from build123d import *

# Parameters (mm, degrees)
EXTRUDE_1_DEPTH     = 2
CUT_EXTRUDE_1_DEPTH = 15.604642381
EXTRUDE_START       = -1.63
EXTRUDE_2_DEPTH     = 1.63
CUT_EXTRUDE_2_DEPTH = 1.2
CUT_EXTRUDE_3_DEPTH = 0.37
FILLET_3_R          = 1.2


with BuildPart() as part:
    # 草图1 → 凸台-拉伸1 (new body)
    with BuildSketch(Plane(origin=(0, 0, 0), x_dir=(-1, 0, 0), z_dir=(0, 1, 0))):
        with BuildLine():
            Line((7.77, 10.437594514), (-7.77, 10.437594514))
            ThreePointArc((-7.77, 10.437594514), (-9.359289322, 9.779289322), (-10.017594514, 8.19))
            Line((-10.017594514, 8.19), (-10.017594514, -8.19))
            ThreePointArc((-10.017594514, -8.19), (-9.359289322, -9.779289322), (-7.77, -10.437594514))
            Line((-7.77, -10.437594514), (7.77, -10.437594514))
            ThreePointArc((7.77, -10.437594514), (9.359289322, -9.779289322), (10.017594514, -8.19))
            Line((10.017594514, -8.19), (10.017594514, 8.19))
            ThreePointArc((10.017594514, 8.19), (9.359289322, 9.779289322), (7.77, 10.437594514))
        make_face()
    extrude(amount=EXTRUDE_1_DEPTH)

    # 草图3 → 切除-拉伸1 (cut, through all)
    with BuildSketch(Plane(origin=(0, 2, 0), x_dir=(1, 0, 0), z_dir=(0, 1, 0))):
        with BuildLine():
            Line((3.175, 8.940777212), (-3.175, 8.940777212))
            ThreePointArc((-3.175, 8.940777212), (-4.200304833, 8.516082045), (-4.625, 7.490777212))
            Line((-4.625, 7.490777212), (-4.625, 6.930777212))
            ThreePointArc((-4.625, 6.930777212), (-4.200304833, 5.90547238), (-3.175, 5.480777212))
            Line((-3.175, 5.480777212), (3.175, 5.480777212))
            ThreePointArc((3.175, 5.480777212), (4.200304833, 5.90547238), (4.625, 6.930777212))
            Line((4.625, 6.930777212), (4.625, 7.490777212))
            ThreePointArc((4.625, 7.490777212), (4.200304833, 8.516082045), (3.175, 8.940777212))
        make_face()
    extrude(amount=-CUT_EXTRUDE_1_DEPTH, mode=Mode.SUBTRACT)

    # 草图4 → 凸台-拉伸2 (add)
    with BuildSketch(Plane.XZ.offset(EXTRUDE_START)):
        with BuildLine():
            Line((-4.625, -7.490777212), (-4.625, -6.930777212))
            ThreePointArc((-4.625, -6.930777212), (-4.200304833, -5.90547238), (-3.175, -5.480777212))
            Line((-3.175, -5.480777212), (3.175, -5.480777212))
            ThreePointArc((3.175, -5.480777212), (4.200304833, -5.90547238), (4.625, -6.930777212))
            Line((4.625, -6.930777212), (4.625, -7.490777212))
            ThreePointArc((4.625, -7.490777212), (4.200304833, -8.516082045), (3.175, -8.940777212))
            Line((3.175, -8.940777212), (-3.175, -8.940777212))
            ThreePointArc((-3.175, -8.940777212), (-4.200304833, -8.516082045), (-4.625, -7.490777212))
        make_face()
        with BuildLine():
            Line((3.175, -8.540777212), (-3.175, -8.540777212))
            ThreePointArc((-3.175, -8.540777212), (-3.91746212, -8.233239333), (-4.225, -7.490777212))
            Line((-4.225, -7.490777212), (-4.225, -6.930777212))
            ThreePointArc((-4.225, -6.930777212), (-3.91746212, -6.188315092), (-3.175, -5.880777212))
            Line((-3.175, -5.880777212), (3.175, -5.880777212))
            ThreePointArc((3.175, -5.880777212), (3.91746212, -6.188315092), (4.225, -6.930777212))
            Line((4.225, -6.930777212), (4.225, -7.490777212))
            ThreePointArc((4.225, -7.490777212), (3.91746212, -8.233239333), (3.175, -8.540777212))
        make_face(mode=Mode.SUBTRACT)
    extrude(amount=EXTRUDE_2_DEPTH)

    # 草图5 → 切除-拉伸2 (cut)
    with BuildSketch(Plane(origin=(0, 2, 0), x_dir=(1, 0, 0), z_dir=(0, 1, 0))):
        with BuildLine():
            Line((9.417594514, 4.880777212), (-9.417594514, 4.880777212))
            Line((-9.417594514, 4.880777212), (-9.417594514, -8.19))
            ThreePointArc((-9.417594514, -8.19), (-8.935025253, -9.355025253), (-7.77, -9.837594514))
            Line((-7.77, -9.837594514), (7.77, -9.837594514))
            ThreePointArc((7.77, -9.837594514), (8.935025253, -9.355025253), (9.417594514, -8.19))
            Line((9.417594514, -8.19), (9.417594514, 4.880777212))
        make_face()
    extrude(amount=-CUT_EXTRUDE_2_DEPTH, mode=Mode.SUBTRACT)

    # 草图7 → 切除-拉伸3 (cut)
    with BuildSketch(Plane(origin=(0, 2, 0), x_dir=(1, 0, 0), z_dir=(0, 1, 0))):
        with BuildLine():
            Line((9.417594514, 8.19), (9.417594514, 4.880777212))
            Line((9.417594514, 4.880777212), (-9.417594514, 4.880777212))
            Line((-9.417594514, 4.880777212), (-9.417594514, 8.19))
            ThreePointArc((-9.417594514, 8.19), (-8.935025253, 9.355025253), (-7.77, 9.837594514))
            Line((-7.77, 9.837594514), (7.77, 9.837594514))
            ThreePointArc((7.77, 9.837594514), (8.935025253, 9.355025253), (9.417594514, 8.19))
        make_face()
    extrude(amount=-CUT_EXTRUDE_3_DEPTH, mode=Mode.SUBTRACT)

    # 圆角3
    fillet_3_edges = [part.edges().sort_by_distance(p)[0] for p in [
        (9.417594514, 1.215, -4.880777212),
        (-9.417594514, 1.215, -4.880777212),
    ]]
    fillet(fillet_3_edges, radius=FILLET_3_R)


solid = part.part
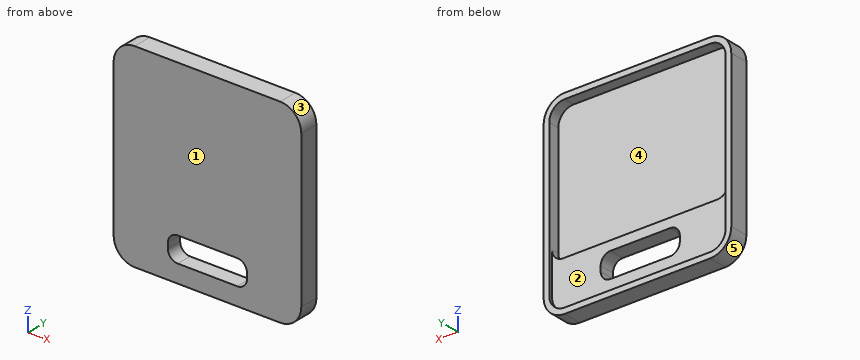
Work out the finished part from the listing and answer in its coordinate system (mm). Face numbers are marked on the shaded views. A direction names the side the tool comes from. Give positions to 0.01 mm unless a question says otherwise; leave off trailing zeros. Loops run counter-clockwise (first coordinate to the right, second up) from the corner with the lowest first, then second, coordinate; pieces in that order, holes last. Notation, with made-up numbers: (32.25, -14.5) - (45.25, -14.5) arc R20 ccw to (45.25, 1.5) - close; hole circle Ø6 at (8.5, 75). An arc over 180 degrees is marked (long way). Answer in a Markdown table with one row per item.
(1) Section C-C (z = -7.75) is taken. Give the vertices of the cut face in (x, y), and give its area (3 significant figures).
Results list:
| item | result |
|---|---|
| outline | (-10.02, 0) - (-4.19, 0) - (-4.19, 1.63) - (-9.42, 1.63) - (-9.42, 2) - (-10.02, 2) - close; (4.19, 0) - (10.02, 0) - (10.02, 2) - (9.42, 2) - (9.42, 1.63) - (4.19, 1.63) - close |
| area | 19.4 mm² |
(2) Section B-B (x = -1) is taken. Give the vertices of the cut face in (y, z).
Results list:
| item | result |
|---|---|
| outline | (0, -10.44) - (2, -10.44) - (2, -9.84) - (1.63, -9.84) - (1.63, -8.54) - (0, -8.54) - close; (0, -5.88) - (1.63, -5.88) - (1.63, -4.88) - (0.8, -4.88) - (0.8, 9.84) - (2, 9.84) - (2, 10.44) - (0, 10.44) - close |
(3) Consider L1, parallel to Z at x = -0.5, y = 1.15; L2, parallel to Z at x = -3, y = 0.65; L3, parallel to Z at x = 4.5, y = 1.3. Determine where each line is inside the solid, lowest interval first. Write a range as [from, to].
Results list:
| item | result |
|---|---|
| L1 | z = [-10.44, -8.54], [-5.88, -4.88], [9.84, 10.44] |
| L2 | z = [-10.44, -8.54], [-5.88, 10.44] |
| L3 | z = [-10.44, -4.88], [9.84, 10.44] |
(4) Section D-D (x = -6.5) is taken. Give the vertices of the cut face in (y, z), and give its area (3 significant figures).
Results list:
| item | result |
|---|---|
| outline | (0, -10.44) - (2, -10.44) - (2, -9.84) - (1.63, -9.84) - (1.63, -4.88) - (0.8, -4.88) - (0.8, 9.84) - (2, 9.84) - (2, 10.44) - (0, 10.44) - close |
| area | 22.3 mm² |
(5) A tool of negligible diameter and unlimited length cuts with its end or side. For the marked faces 1 and 2, from which of +Z, -Z, +X, -X, +Y, -Y can it reach the whole face along a straight path? Write none if from no direction.
Results list:
| item | result |
|---|---|
| face 1 | +Z, -Z, +X, -X, -Y |
| face 2 | +Y |
(6) Section A-A (y = 1.2) is taken. Give the vertices of the cut face in (x, z) (3 decimals).
Results list:
| item | result |
|---|---|
| outline | (-10.018, -8.19) arc R2.248 ccw to (-7.77, -10.438) - (7.77, -10.438) arc R2.248 ccw to (10.018, -8.19) - (10.018, 8.19) arc R2.248 ccw to (7.77, 10.438) - (-7.77, 10.438) arc R2.248 ccw to (-10.018, 8.19) - close; hole (-9.418, -3.681) arc R1.2 ccw to (-8.218, -4.881) - (8.218, -4.881) arc R1.2 ccw to (9.418, -3.681) - (9.418, 8.19) arc R1.648 ccw to (7.77, 9.838) - (-7.77, 9.838) arc R1.648 ccw to (-9.418, 8.19) - close; hole (-4.225, -7.491) arc R1.05 ccw to (-3.175, -8.541) - (3.175, -8.541) arc R1.05 ccw to (4.225, -7.491) - (4.225, -6.931) arc R1.05 ccw to (3.175, -5.881) - (-3.175, -5.881) arc R1.05 ccw to (-4.225, -6.931) - close |
(7) For a pull along X with two mould halves and no side action, classify the marked faces 3, 4 and 5 as pulls with the +X half, pulls with the -X half, needs draft (parallel to the pull), parting line crosses it, or undercut.
Results list:
| item | result |
|---|---|
| face 3 | pulls with the +X half |
| face 4 | undercut |
| face 5 | pulls with the -X half |
(8) Flat-ended cylindrical pins translate along their axes: pin 1 Ø4 at (x, z) = (-7, 1.5) entering from +Y; pin 2 Ø3 at (x, z) = (1, -5.5) entering from +Y. Find the tip coordinate at first contact, or state that the pin passes through.
Results list:
| item | result |
|---|---|
| pin 1 | stops at y = 0.8 |
| pin 2 | stops at y = 1.63 |
